Autodesk Inventor part; units mm, degrees
ref_plane "YZ Plane" through (0, 0, 0) normal (1, 0, 0) x (0, 1, 0)
ref_plane "XZ Plane" through (0, 0, 0) normal (0, 1, 0) x (-1, 0, 0)
ref_plane "XY Plane" through (0, 0, 0) normal (0, 0, 1) x (1, 0, 0)
sketch "Sketch1" plane through (0, 0, 0) normal (0, 0, 1) x (1, 0, 0)
  line L0 (-3.2079, 5.5563) -> (3.2079, 5.5563)
  line L1 (3.2079, 5.5563) -> (6.4158, 0)
  line L2 (6.4158, 0) -> (3.2079, -5.5563)
  line L3 (3.2079, -5.5563) -> (-3.2079, -5.5562)
  line L4 (-3.2079, -5.5562) -> (-6.4158, 0)
  line L5 (-6.4158, 0) -> (-3.2079, 5.5563)
  point P0 (0, 0)
  point P1 (0, 0)
  dimension "d0" = 11.1125
extrude "Extrusion1" add sketch "Sketch1" along normal blind 6.35
sketch "Sketch3" plane through (0, 0, 6.35) normal (0, 0, 1) x (1, 0, 0)
  circle A0 centre (0, 0) radius 5.08
  dimension "d28" = 10.16
extrude "Extrusion2" add sketch "Sketch3" along normal blind 1.5875
sketch "Sketch8" plane through (0, 0, 7.9375) normal (0, 0, 1) x (1, 0, 0)
  circle A0 centre (0, 0) radius 5.08
  circle A1 centre (0, 0) radius 3.175
  dimension "d29" = 6.35
sketch "Sketch9" plane through (0, 0, 0) normal (0, 0, -1) x (-1, 0, 0)
  point P0 (0, 0)
hole "Hole2" at (0, 0, 0) direction (0, 0, 1) diameter 4.9784 end through all
sketch "Sketch10" plane through (0, 0, 0) normal (0, 1, 0) x (-1, 0, 0)
  line L0 (-6.4158, 6.35) -> (-3.2079, 6.35)
  line L1 (-3.2079, 0) -> (-3.2079, 6.35)
  line L2 (-6.4158, 0) -> (-3.2079, 0)
  line L3 (-6.4158, 0) -> (-6.4158, 6.35)
  line L4 (0, 0) -> (0, 6.9243)
  arc A0 (-4.572, 6.35) -> (-6.4158, 5.1517) centre (-4.572, 4.3324) ccw
  line L5 (-6.4158, 5.1517) -> (-6.4158, 6.35)
  line L6 (-4.572, 6.35) -> (-6.4158, 6.35)
  dimension "d24" = 4.572
revolve "Revolution2" cut sketch "Sketch10" angle 360 about axis through (0, 0, 0) along (0, 0, 1) contours L0 A0 L3
fillet "Fillet1" radius 0.508 12 edges at (-3.2079, -5.5562, 2.5758) (3.2079, -5.5563, 2.5758) (6.4158, 0, 2.5758) (3.2079, 5.5563, 2.5758) (-6.4158, 0, 2.5758) (-3.2079, 5.5563, 2.5758) (0, 5.5563, 0) (4.8119, 2.7781, 0) (4.8119, -2.7781, 0) (0, -5.5563, 0) (-4.8119, -2.7781, 0) (-4.8119, 2.7781, 0)
fillet "Fillet2" radius 0.508 1 edges at (-5.08, 0, 7.9375)
extrude "Extrusion4" cut sketch "Sketch8" against normal blind 0.254 contours A1
properties part number "14-20 regular lock nut" material "Steel"
The listing builds one solid part. Answer for the finished solid, in the listing's coordinates (mm). A direction names the side the tool comes from. Coordinates: 2 decimals unless noted, no trailing zeros. Loops run counter-clockwise (first coordinate to the right, second up) from the corner with the lowest first, then second, coordinate; pieces in that order, holes last. Notation, with made-up numbers: M 41,36.25 L 45,36.25 A19 ccw 45,72.25 Z; hole C 87.5,-15 d8. An arc over 180 degrees is marked long. Answer in a Markdown table with one row per item.
1) Find section A-A (z = 4). Determine the outline of the cut face in (x, y).
Answers below:
| item | result |
|---|---|
| outline | M -6.27,-0.25 L -3.35,-5.3 A0.51 ccw -2.91,-5.56 L 2.91,-5.56 A0.51 ccw 3.35,-5.3 L 6.27,-0.25 A0.51 ccw 6.27,0.25 L 3.35,5.3 A0.51 ccw 2.91,5.56 L -2.91,5.56 A0.51 ccw -3.35,5.3 L -6.27,0.25 A0.51 ccw Z; hole C 0,0 d4.98 |
2) Find the intervals of material crossed by probe 1 along X at (y, z) = (0, 4.75); probe 2 along Y at (x, z) = (0, 2.25); probe 3 along Y at (x, z) = (-3.5, 4.75), in increasing order.
Answers below:
| item | result |
|---|---|
| probe 1 | -6.34 to -2.49, 2.49 to 6.34 |
| probe 2 | -5.56 to -2.49, 2.49 to 5.56 |
| probe 3 | -5.05 to 5.05 |
3) Which of the six approach directions +Z, -Z, +X, -X, +Y, -Y give full straight-line access (tool end or side, diameter ignored) to faces 1 (the flat face through (0, 5.556, 3)), 2 (the cylindrical face through (-0.661, -5.037, 6.882))?
Answers below:
| item | result |
|---|---|
| face 1 | +Z, -Z, +X, -X, +Y |
| face 2 | +Z |
4) Find section B-B (z = 6.75). Determine the outline of the cut face in (x, y).
Answers below:
| item | result |
|---|---|
| outline | C 0,0 d10.16; hole C 0,0 d4.98 |
5) Given pin 1 (3 mm diameter, centred on x = -1, y = -1.5, fed in from -Z); pin 2 (1 mm diameter, centred on y = -2.5, z = 4.5, fed in from -X), each flat-ended and moving along its own axis, determine where each tip first touches the part or whether it passes through.
Answers below:
| item | result |
|---|---|
| pin 1 | z = 0 |
| pin 2 | x = -5.26 |
6) Determine the mould class of faces 3 (the cylindrical face through (-4.707, 2.67, 0.153)), 4 (the cylindrical face through (-0.748, 2.374, 3.896)), 5 (the flat face through (-4.8, -2.8, 3.3)) for opening direction Y: released by +Y, released by -Y, zero draft, split by the parting line, or undercut.
Answers below:
| item | result |
|---|---|
| face 3 | released by +Y |
| face 4 | undercut |
| face 5 | released by -Y |
